Part model, mm, in its own coordinate system. A direction names the side the tool comes from. Coordinates: 2 decimals unless noted, no trailing zeros. Order: outer loops, then holes, each group sorted by start corner. A loop starts at its lowest first (then second) coordinate and runs counter-clockwise, first axis right, second up. Notation, with made-up numbers: (33.5, 9.5) - (89.5, 9.5) arc R21 cw to (89.5, 13.5) - close; hole circle Ø4 at (-16, -23.75). An arc over 180 degrees is marked (long way). Use a Markdown table: item, result. Add a question column.
1) Saw through at C-C on z = 0. List the corners of the cut face in (x, y), then the cut area to 3 significant figures.
2) Two-plate mould, pull along Z, no slides. Class faces 1 (the face through (0, 2, 3.2)), 2 (the face through (-4, 2, 1)), 3 (the face through (-4, 0, 0)): +Z half, -Z half, draft (parallel to the pull), parting line (faces both ways), or undercut.
3) Wall check: L1, parallel to Y at x = 2.5, z = -1.5; L2, parallel to X at y = 1.35, z = 3.5; L3, parallel to Z at x = -1, y = 2.4. Give the ranges that are in metal, low to high. Write a range as [from, to].
4) Tool access for faces 4 (the face through (0, 2, -3.2)), 5 (the face through (3.2, 2, 0)), 6 (the face through (2, 2, 4)), 7 (the face through (4, 2, -1)): list every direction of +Z, -Z, +X, -X, +Y, -Y with a clear straight run to the whole face (end or side of a thin tool).
5) Saw through at B-B on x = 0. List the corners of the cut face in (y, z), then the cut area to 3 significant figures.
6) Saw through at A-A on y = 2.2. List the corners of the cut face in (x, z), then the cut area to 3 significant figures.
7) Drop flat-ended pins along their axis: P1, Ø3, axis at x = -0.5, y = 4, coming from the +Z side; P2, Ø1.2, axis at y = 2, z = -3.5, coming from the -X side; P3, Ø1.5, axis at x = -2, y = 1.5, coming from the -Z side; P4, Ø0.6, axis at y = 1.5, z = -4, coming from the +X side. Give the stop position or say it passes through.
```python
from build123d import *

# Parameters (mm, degrees)
BOSS_EXTRUDE1_DEPTH   = 5
BOSS_EXTRUDE1_2_DEPTH = 5
BOSS_EXTRUDE1_3_DEPTH = 5
BOSS_EXTRUDE1_4_DEPTH = 5
BOSS_EXTRUDE2_START   = -1
SKETCH2_R             = 4.75
SKETCH2_R_2           = 2.313447094
BOSS_EXTRUDE2_DEPTH   = 1
CHAMFER1_SIZE         = 0.5


with BuildPart() as part:
    # Sketch1 → Boss-Extrude1 (new body)
    with BuildSketch(Plane(origin=(0, 0, 0), x_dir=(1, 0, 0), z_dir=(0, 1, 0))):
        with BuildLine():
            Line((3.2, -1), (3.2, 1))
            Line((3.2, 1), (4.643543905, 1))
            ThreePointArc((4.643543905, 1), (4.75, 0), (4.643543905, -1))
            Line((4.643543905, -1), (3.2, -1))
        make_face()
    extrude(amount=BOSS_EXTRUDE1_DEPTH)



with BuildPart() as body_2:
    # Sketch1 → Boss-Extrude1 2 (new body)
    with BuildSketch(Plane(origin=(0, 0, 0), x_dir=(1, 0, 0), z_dir=(0, 1, 0))):
        with BuildLine():
            Line((-4.643543905, -1), (-3.2, -1))
            Line((-3.2, -1), (-3.2, 1))
            Line((-3.2, 1), (-4.643543905, 1))
            ThreePointArc((-4.643543905, 1), (-4.75, 0), (-4.643543905, -1))
        make_face()
    extrude(amount=BOSS_EXTRUDE1_2_DEPTH)


with BuildPart() as body_3:
    # Sketch1 → Boss-Extrude1 3 (new body)
    with BuildSketch(Plane(origin=(0, 0, 0), x_dir=(1, 0, 0), z_dir=(0, 1, 0))):
        with BuildLine():
            Line((-2, -4.308421985), (-2, -3.2))
            Line((-2, -3.2), (2, -3.2))
            Line((2, -3.2), (2, -4.308421985))
            ThreePointArc((2, -4.308421985), (0, -4.75), (-2, -4.308421985))
        make_face()
    extrude(amount=BOSS_EXTRUDE1_3_DEPTH)


with BuildPart() as body_4:
    # Sketch1 → Boss-Extrude1 4 (new body)
    with BuildSketch(Plane(origin=(0, 0, 0), x_dir=(1, 0, 0), z_dir=(0, 1, 0))):
        with BuildLine():
            Line((-2, 4.308421985), (-2, 3.2))
            Line((-2, 3.2), (2, 3.2))
            Line((2, 3.2), (2, 4.308421985))
            ThreePointArc((2, 4.308421985), (0, 4.75), (-2, 4.308421985))
        make_face()
    extrude(amount=BOSS_EXTRUDE1_4_DEPTH)


with BuildPart() as part_1:
    add(part.part)

    add(body_2.part)  # Boss-Extrude2 merges body 2

    add(body_3.part)  # Boss-Extrude2 merges body 3

    add(body_4.part)  # Boss-Extrude2 merges body 4
    # Sketch2 → Boss-Extrude2 (add)
    with BuildSketch(Plane(origin=(0, 5, 0), x_dir=(1, 0, 0), z_dir=(0, 1, 0)).offset(BOSS_EXTRUDE2_START)):
        with Locations(Location((0, 0, 0), (0, 0, 90))):
            Circle(SKETCH2_R)
        with Locations(Location((0, 0, 0), (0, 0, 270))):
            Circle(SKETCH2_R_2, mode=Mode.SUBTRACT)
    extrude(amount=BOSS_EXTRUDE2_DEPTH)

    # Chamfer1
    chamfer1_edges = [part_1.edges().sort_by_distance(p)[0] for p in [
        (-1.024083876, 5, -4.63829195),
    ]]
    chamfer(chamfer1_edges, length=CHAMFER1_SIZE)


solid = part_1.part
```
Results are:
| question | item | result |
|---|---|---|
| 1 | outline | (-4.75, 0) - (-3.2, 0) - (-3.2, 4) - (-2.31, 4) - (-2.31, 5) - (-4.25, 5) - (-4.75, 4.5) - close; (2.31, 4) - (3.2, 4) - (3.2, 0) - (4.75, 0) - (4.75, 4.5) - (4.25, 5) - (2.31, 5) - close |
| 1 | area | 17.0 mm2 |
| 2 | face 1 | undercut |
| 2 | face 2 | +Z half |
| 2 | face 3 | draft |
| 3 | L1 | [4, 5] |
| 3 | L2 | [-2, 2] |
| 3 | L3 | [-4.64, -3.2], [3.2, 4.64] |
| 4 | face 4 | +X, -X, -Y |
| 4 | face 5 | +Z, -Z, -Y |
| 4 | face 6 | +Z, -Z, +X, -Y |
| 4 | face 7 | -Z, +X, -X, -Y |
| 5 | outline | (0, -4.75) - (4.5, -4.75) - (5, -4.25) - (5, -2.31) - (4, -2.31) - (4, -3.2) - (0, -3.2) - close; (0, 3.2) - (4, 3.2) - (4, 2.31) - (5, 2.31) - (5, 4.25) - (4.5, 4.75) - (0, 4.75) - close |
| 5 | area | 17.0 mm2 |
| 6 | outline | (-4.64, -1) - (-3.2, -1) - (-3.2, 1) - (-4.64, 1) arc R4.75 ccw to start; (-2, -4.31) arc R4.75 ccw to (2, -4.31) - (2, -3.2) - (-2, -3.2) - close; (-2, 3.2) - (2, 3.2) - (2, 4.31) arc R4.75 ccw to (-2, 4.31) - close; (3.2, -1) - (4.64, -1) arc R4.75 ccw to (4.64, 1) - (3.2, 1) - close |
| 6 | area | 17.3 mm2 |
| 7 | P1 | z = 4.75 |
| 7 | P2 | x = -2 |
| 7 | P3 | z = -4.58 |
| 7 | P4 | x = 2 |
